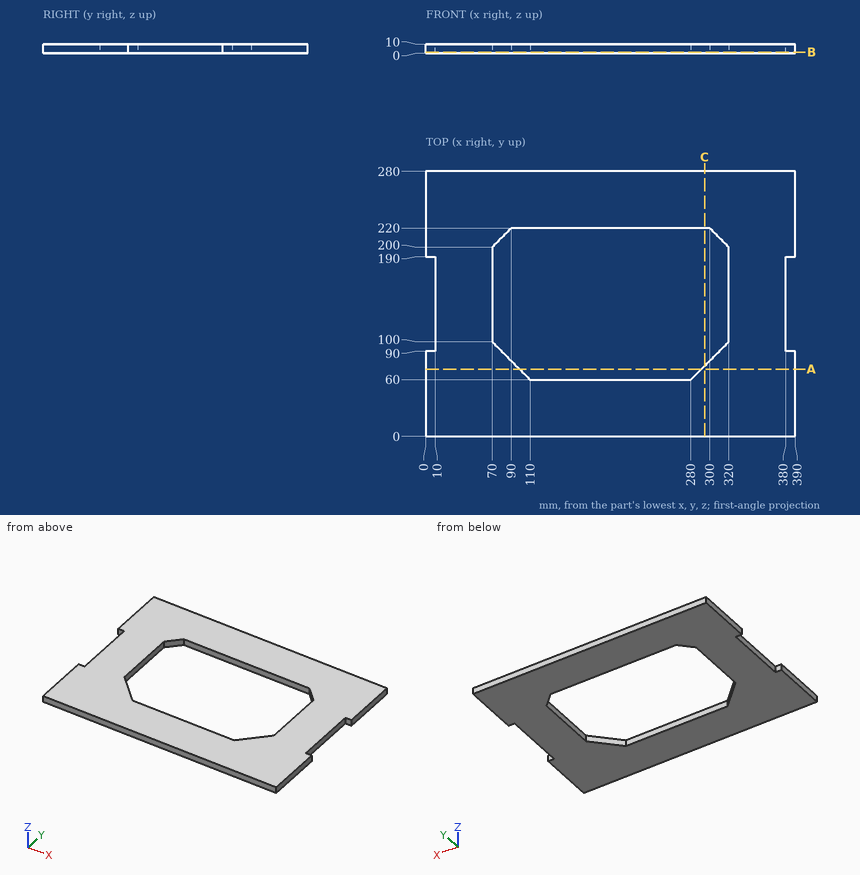
Study the drawing (mm; zero at the part's minimum x, y, z) and answer. Round coordinates to 2 decimals unless told otherwise and drop trailing zeros. Loops run counter-clockwise (first coordinate to the right, second up) from the corner with the lowest first, then second, coordinate; pieces in that order, holes last. Notation, with made-up numbers: (88, -0.5) -> (92, -0.5) arc R28 ccw to (92, 22.5) -> close; hole circle Ø9 at (64.5, 65.25). An arc over 180 degrees is marked (long way). Use one line per item in the form item = value.
1. The part is cut by section B-B on z = 1.5. Determine the outline of the cut face in (x, y).
Answer key:
outline = (0, 0) -> (390, 0) -> (390, 90) -> (380, 90) -> (380, 190) -> (390, 190) -> (390, 280) -> (0, 280) -> (0, 190) -> (10, 190) -> (10, 90) -> (0, 90) -> close; hole (70, 100) -> (110, 60) -> (280, 60) -> (320, 100) -> (320, 200) -> (300, 220) -> (90, 220) -> (70, 200) -> close
2. A flat-ended cylindrical pin translates along its axis: pin 1 Ø3 at (y, z) = (139.5, 5.5) entering from +X. Find the tip coordinate at first contact, or state that the pin passes through.
Answer key:
pin_1 = 380
3. The part is cut by section A-A on y = 71. Determine the outline of the cut face in (x, z).
Answer key:
outline = (0, 0) -> (99, 0) -> (99, 10) -> (0, 10) -> close; (291, 0) -> (390, 0) -> (390, 10) -> (291, 10) -> close
4. The part is cut by section C-C on x = 294.5. Determine the outline of the cut face in (y, z), and give its area (4 significant figures).
Answer key:
outline = (0, 0) -> (74.5, 0) -> (74.5, 10) -> (0, 10) -> close; (220, 0) -> (280, 0) -> (280, 10) -> (220, 10) -> close
area = 1,345 mm²
5. Find the intervals of material crossed by probe 1 along Y at (x, z) = (167, 4); probe 2 along Y at (x, z) = (100, 7); probe 3 along X at (y, z) = (122, 8.75), in increasing order. Write a range as [from, to].
Answer key:
probe_1 = [0, 60], [220, 280]
probe_2 = [0, 70], [220, 280]
probe_3 = [10, 70], [320, 380]
